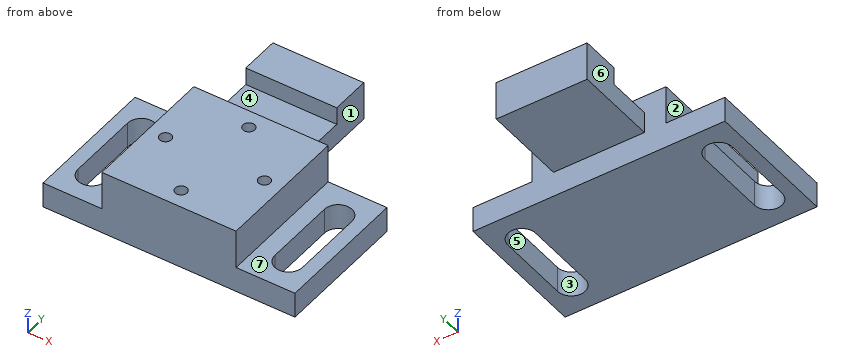
from build123d import *

# Parameters (mm, degrees)
SKETCH1_W           = 64
SKETCH1_H           = 34.1
BOSS_EXTRUDE1_DEPTH = 6.5
BOSS_EXTRUDE2_DEPTH = 9.9
SKETCH4_W           = 23.11
SKETCH4_H           = 11.2
CUT_EXTRUDE1_DEPTH  = 4.5
CUT_EXTRUDE2_DEPTH  = 7.5
SKETCH7_R           = 1.5
CUT_EXTRUDE3_DEPTH  = 10


with BuildPart() as part:
    # Sketch1 → Boss-Extrude1 (new body)
    with BuildSketch(Plane.XY):
        Rectangle(SKETCH1_W, SKETCH1_H)
    extrude(amount=BOSS_EXTRUDE1_DEPTH)

    # Sketch2 → Boss-Extrude2 (add)
    with BuildSketch(Plane.XY.offset(6.5)):
        Polygon((-17.05, 17.05), (-11.555, 17.05), (-11.555, 38.25), (11.555, 38.25), (11.555, 17.05), (17.05, 17.05), (17.05, -17.05), (-17.05, -17.05), align=None)
    extrude(amount=BOSS_EXTRUDE2_DEPTH)

    # Sketch4 → Cut-Extrude1 (cut)
    with BuildSketch(Plane.XY.offset(16.4)):
        with Locations((0, 22.65)):
            Rectangle(SKETCH4_W, SKETCH4_H)
    extrude(amount=-CUT_EXTRUDE1_DEPTH, mode=Mode.SUBTRACT)

    # Sketch6 → Cut-Extrude2 (cut, through all)
    with BuildSketch(Plane.XY.offset(6.5)):
        with BuildLine():
            Line((-21.5, 9.178681579), (-21.5, -9.178681579))
            ThreePointArc((-21.5, -9.178681579), (-25, -12.678681579), (-28.5, -9.178681579))
            Line((-28.5, -9.178681579), (-28.5, 9.178681579))
            ThreePointArc((-28.5, 9.178681579), (-25, 12.678681579), (-21.5, 9.178681579))
        make_face()
    cut_extrude2 = extrude(amount=-CUT_EXTRUDE2_DEPTH, mode=Mode.SUBTRACT)

    # Mirror1: Cut-Extrude2 across plane
    add(cut_extrude2.mirror(Plane(origin=(0, 0, 0), x_dir=(0, 0, 1), z_dir=(1, 0, 0))), mode=Mode.SUBTRACT)

    # Sketch7 → Cut-Extrude3 (cut)
    with BuildSketch(Plane.XY.offset(16.4)):
        with Locations((-12.55, 0)):
            Circle(SKETCH7_R)
        with Locations((12.55, 0)):
            Circle(SKETCH7_R)
        with Locations((0, 12.55)):
            Circle(SKETCH7_R)
        with Locations((0, -12.55)):
            Circle(SKETCH7_R)
    extrude(amount=-CUT_EXTRUDE3_DEPTH, mode=Mode.SUBTRACT)


solid = part.part
Can you work these out from the model? Positions are in its coordinate system, mm. Face numbers are marked on the shaded views. A direction names the side the tool comes from. Coordinates: 2 decimals unless noted, no trailing zeros. Write each loop counter-clockwise with the first axis right and the second up, starting at its lowest first coordinate (ties: lowest second). Pieces come first, ordered by that corner, then holes. Notation, with made-up numbers: (-24.5, 84.25) -> (11.5, 84.25) arc R29 ccw to (11.5, 123.25) -> close; hole circle Ø5 at (37, -9.5). An arc over 180 degrees is marked (long way). Answer as CSV lines item,"result".
1) If we section it at D-D on y = 15.5: Please give me the cut outline in (x, z), then the cut area to 3 significant figures.
Check result:
outline,"(-32, 0) -> (32, 0) -> (32, 6.5) -> (17.05, 6.5) -> (17.05, 16.4) -> (-17.05, 16.4) -> (-17.05, 6.5) -> (-32, 6.5) -> close"
area,"754 mm²"
2) If I drill on line 1 (X direction, y = 1, z = 5.25); line 2 (Y direction, x = 0, z = 12.5); line 3 (Y direction, x = -12.55, z = 14.25), over which ranges is the centre line in solid material (lowest first)? Write a range as from..to.
Check result:
line 1,"-32..-28.5, -21.5..21.5, 28.5..32"
line 2,"-17.05..-14.05, -11.05..11.05, 14.05..17.05, 28.25..38.25"
line 3,"-17.05..-1.5, 1.5..17.05"
3) On a 3-axis mill with a long thin cutter (end or side, diameter ignored), from which of +Z, -Z, +X, -X, +Y, -Y can I reach the whole of each face in a straight line? I mean the marked faces 4, 5, 6 and 7. Say none if no direction works.
Check result:
face 4,"+Z, +X, -X"
face 5,"+Z, -Z"
face 6,"+Z, -Z, -X, +Y"
face 7,"+Z, +X, +Y, -Y"
4) Will these pins go through, and if not, where does the flat tip stop? P1, Ø17, axis at x = -4, y = 31, coming from the -Z side; P2, Ø5, axis at y = 31, z = 10.5, coming from the -X side (3 decimals); P3, Ø0.9, axis at x = -12.5, y = -0.5, coming from the +Z side.
Check result:
P1,"z = 6.5"
P2,"x = -11.555"
P3,"z = 6.4"
5) If we section it at C-C on x = 0: Please give me the cut outline in (y, z), then the cut area to 3 significant figures.
Check result:
outline,"(-17.05, 0) -> (17.05, 0) -> (17.05, 6.5) -> (38.25, 6.5) -> (38.25, 16.4) -> (28.25, 16.4) -> (28.25, 11.9) -> (17.05, 11.9) -> (17.05, 16.4) -> (14.05, 16.4) -> (14.05, 6.4) -> (11.05, 6.4) -> (11.05, 16.4) -> (-11.05, 16.4) -> (-11.05, 6.4) -> (-14.05, 6.4) -> (-14.05, 16.4) -> (-17.05, 16.4) -> close"
area,"659 mm²"
6) If we section it at B-B on z = 2.5: Please give me the cut outline in (x, y).
Check result:
outline,"(-32, -17.05) -> (32, -17.05) -> (32, 17.05) -> (-32, 17.05) -> close; hole (-28.5, -9.18) arc R3.5 ccw to (-21.5, -9.18) -> (-21.5, 9.18) arc R3.5 ccw to (-28.5, 9.18) -> close; hole (21.5, -9.18) arc R3.5 ccw to (28.5, -9.18) -> (28.5, 9.18) arc R3.5 ccw to (21.5, 9.18) -> close"
7) If we section it at A-A on x = 25: Please give me the cut outline in (y, z), then the cut area to 3 significant figures.
Check result:
outline,"(-17.05, 0) -> (-12.68, 0) -> (-12.68, 6.5) -> (-17.05, 6.5) -> close; (12.68, 0) -> (17.05, 0) -> (17.05, 6.5) -> (12.68, 6.5) -> close"
area,"56.8 mm²"
8) If we mould it in two halves opening along X, with no side actions, what happens to the marked faces 1, 2 and 3? For each: +X half, -X half, draft (parallel to the pull), parting line (faces both ways), or undercut.
Check result:
face 1,"+X half"
face 2,"-X half"
face 3,"undercut"
